The drawing under review shows one solid part. Ordinate dimensions are in mm from its lowest x, y, z. Round coordinates to 2 decimals unless told otherwise and drop trailing zeros. Write each loop counter-clockwise with the first axis right and the second up, starting at its lowest first coordinate (ties: lowest second). Pieces come first, ordered by that corner, then holes.
Item 1: Add section C-C (y = 190.5). Give the boundary of the cut face in (x, z), plus the area to 3 significant figures.
Item 2: Draft analysis for pull direction X (two halves, no side actions). For the marked faces 1, 2 and 3, state which applies: +X half, -X half, draft (parallel to the pull), parting line (faces both ways), or undercut.
Item 3: Add section B-B (z = 68). Give the boundary of the cut face in (x, y), plus the area to 4 significant figures.
Item 4: To check wall thickness, follow L1, parallel to X at y = 62.5, z = 68; L2, parallel to Y at x = 71.5, z = 111. State the ranges of each line that lie inside material, in increasing order.
Item 5: Add section A-A (x = 68). Give the boundary of the cut face in (y, z), plus the area to 3 significant figures.
Item 6: Clearance check with flat-ended pins moving along their axes: pin 1 Ø10 at (x, z) = (92.5, 26.5) entering from -Y; pin 2 Ø8.5 at (y, z) = (11, 40) entering from +X; pin 3 Ø8.5 at (y, z) = (29.5, 98) entering from -X. State where each tip first meets the part, or that it passes through.
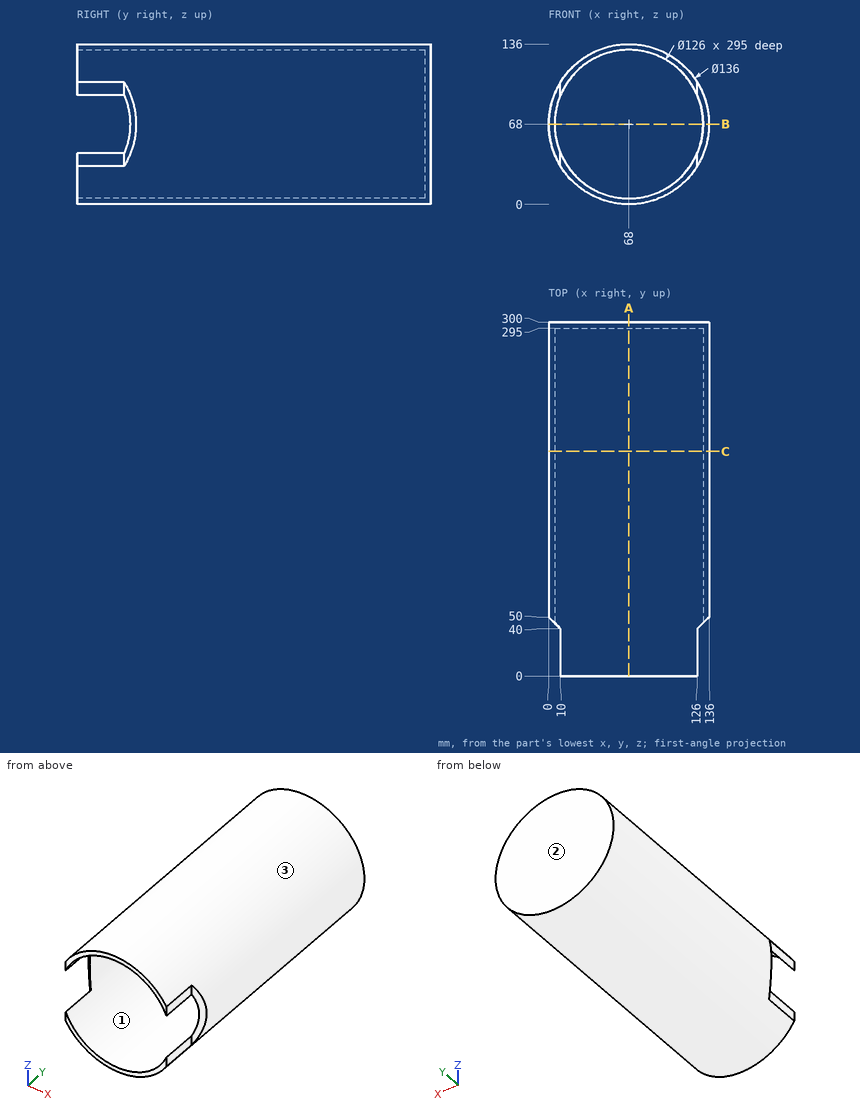
Numbers:
1. outline: circle Ø136 at (68, 68); hole circle Ø126 at (68, 68)
1. area: 2,060 mm2
2. face 1: undercut
2. face 2: draft
2. face 3: parting line
3. outline: (0, 50) - (5, 45) - (5, 295) - (131, 295) - (131, 45) - (136, 50) - (136, 300) - (0, 300) - close
3. area: 3,155 mm2
4. L1: x = 0 to 5, 131 to 136
4. L2: y = 295 to 300
5. outline: (0, 0) - (300, 0) - (300, 136) - (0, 136) - (0, 131) - (295, 131) - (295, 5) - (0, 5) - close
5. area: 3,630 mm2
6. pin 1: stops at y = 295
6. pin 2: stops at x = 126
6. pin 3: stops at x = 10
